Print and shaded views of the part. All mm, measured from the part's lowest x, y and z. A direction names the side the tool comes from. Round coordinates to 2 decimals unless told otherwise and drop trailing zeros. Order: outer loops, then holes, each group sorted by start corner. A loop starts at its lowest first (then second) coordinate and runs counter-clockwise, first axis right, second up. Notation, with made-up numbers: (36, 65.5) - (95, 65.5) arc R9 ccw to (95, 82.5) - close; hole circle Ø5 at (21.5, 70.25). An arc over 180 degrees is marked (long way). Write item = value, one per line. Start each with the question number.
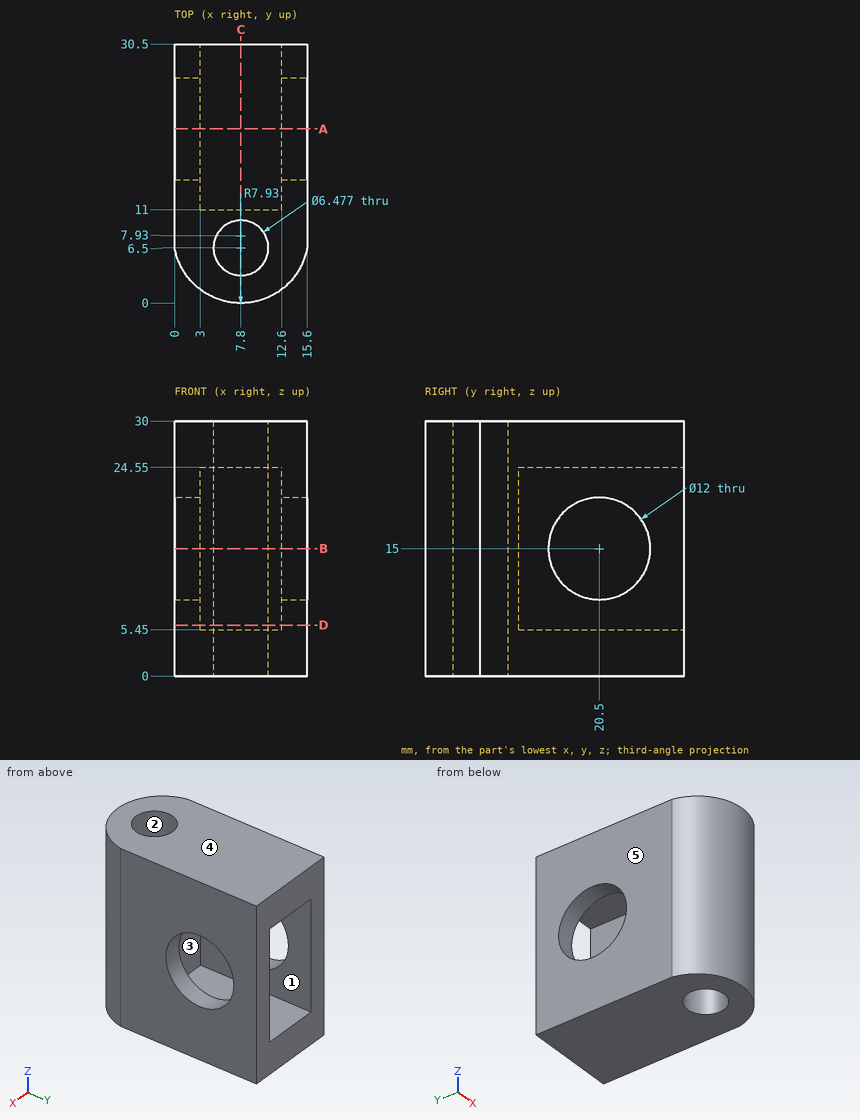
Item 1: Probe L1, parallel to Y at x = 8, z = 10.75; L2, parallel to X at y = 21.5, z = 23; L3, parallel to Z at x = 10.75, y = 25.5. List the from-to ranges inside material, lowest first.
Item 2: Saw through at D-D, the plane z = 6. Give the cut face in (x, y).
Item 3: Saw through at B-B, the plane z = 15. Give the cut face in (x, y).
Item 4: Drop flat-ended pins along their axis: pin 1 (3 mm diameter, centred on x = 8.5, z = 23, fed in from +Y); pin 2 (2 mm diameter, centred on x = 2.5, z = 13, fed in from -Y); pin 3 (1.5 mm diameter, centred on y = 20, z = 20, fed in from -X). Give the stop position or say it passes through.
Item 5: Saw through at A-A, the plane y = 20.5. Give the cut face in (x, z).
Item 6: Saw through at C-C, the plane x = 7.8. Give the cut face in (y, z), then the cut area to 3 significant figures.
Item 7: Which spindle directions (+Z, -Z, +X, -X, +Y, -Y) get a long thin tool onto all of the face, cutting with end or side? Do the marked faces 1 and 2. Say none if no direction does.
Item 8: Mould opens along X. For the marked faces 3, 4 and 5 say: +X half, -X half, draft (parallel to the pull), parting line (faces both ways), or undercut.
Check sheet entries:
q1.L1 = 0 to 3.27, 9.73 to 11
q1.L2 = 0 to 3, 12.6 to 15.6
q1.L3 = 0 to 5.45, 24.55 to 30
q2.outline = (0, 6.5) arc R7.93 ccw to (15.6, 6.5) - (15.6, 30.5) - (12.6, 30.5) - (12.6, 11) - (3, 11) - (3, 30.5) - (0, 30.5) - close; hole circle Ø6.48 at (7.8, 6.5)
q3.outline = (0, 6.5) arc R7.93 ccw to (15.6, 6.5) - (15.6, 14.5) - (12.6, 14.5) - (12.6, 11) - (3, 11) - (3, 14.5) - (0, 14.5) - close; (0, 26.5) - (3, 26.5) - (3, 30.5) - (0, 30.5) - close; (12.6, 26.5) - (15.6, 26.5) - (15.6, 30.5) - (12.6, 30.5) - close; hole circle Ø6.48 at (7.8, 6.5)
q4.pin_1 = 11
q4.pin_2 = 1.27
q4.pin_3 = through
q5.outline = (0, 0) - (15.6, 0) - (15.6, 9) - (12.6, 9) - (12.6, 5.45) - (3, 5.45) - (3, 9) - (0, 9) - close; (0, 21) - (3, 21) - (3, 24.55) - (12.6, 24.55) - (12.6, 21) - (15.6, 21) - (15.6, 30) - (0, 30) - close
q6.outline = (0, 0) - (3.26, 0) - (3.26, 30) - (0, 30) - close; (9.74, 0) - (30.5, 0) - (30.5, 5.45) - (11, 5.45) - (11, 24.55) - (30.5, 24.55) - (30.5, 30) - (9.74, 30) - close
q6.area = 348 mm2
q7.face_1 = +Y
q7.face_2 = +Z, -Z
q8.face_3 = undercut
q8.face_4 = draft
q8.face_5 = -X half
